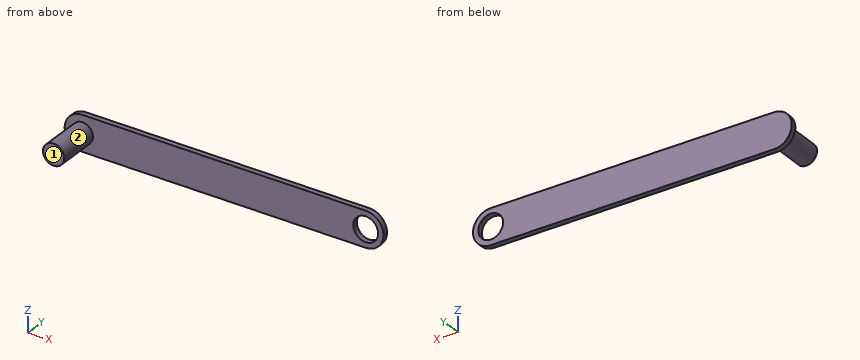
```python
from build123d import *

# Parameters (mm, degrees)
F0_R     = 3.5
F1_DEPTH = 1.5
F2_R     = 3
F3_DEPTH = 12


with BuildPart() as f1:
    # F0 (on Front) → F1 (new body)
    with BuildSketch(Plane.XZ):
        with BuildLine():
            Line((80, 5), (0, 5))
            ThreePointArc((0, 5), (-5, 0), (0, -5))
            Line((0, -5), (80, -5))
            ThreePointArc((80, -5), (85, 0), (80, 5))
        make_face()
        with Locations((80, 0)):
            Circle(F0_R, mode=Mode.SUBTRACT)
    extrude(amount=F1_DEPTH)

    # F2 (on face) → F3 (join)
    with BuildSketch(Plane.XZ.offset(1.5)):
        Circle(F2_R)
    extrude(amount=F3_DEPTH)


solid = f1.part
```
Source: CAD feature listing. Evaluate the final solid. Frame: model axes, mm. Face numbers are marked on the shaded views. Give positions to 0.01 mm unless a question says otherwise; leave off trailing zeros. Order: outer loops, then holes, each group sorted by start corner. A loop starts at its lowest first (then second) coordinate and runs counter-clockwise, first axis right, second up. Notation, with made-up numbers: (23.5, 77.5) -> (68.5, 77.5) arc R24 ccw to (68.5, 91.5) -> close; hole circle Ø8 at (-3.5, -39.75). An arc over 180 degrees is marked (long way). Use a Markdown table: item, result.
Q1. Section A-A (z = 0). Return the cut outline in (x, y), and give its area (4 significant figures).
A:
| item | result |
|---|---|
| outline | (-5, -1.5) -> (-3, -1.5) -> (-3, -13.5) -> (3, -13.5) -> (3, -1.5) -> (76.5, -1.5) -> (76.5, 0) -> (-5, 0) -> close; (83.5, -1.5) -> (85, -1.5) -> (85, 0) -> (83.5, 0) -> close |
| area | 196.5 mm^2 |
Q2. Section B-B (x = 2). Return the cut outline in (y, z).
A:
| item | result |
|---|---|
| outline | (-13.5, -2.24) -> (-1.5, -2.24) -> (-1.5, -5) -> (0, -5) -> (0, 5) -> (-1.5, 5) -> (-1.5, 2.24) -> (-13.5, 2.24) -> close |
Q3. Material intervals for line 1 (Z direction, x = 80, y = -0.8); line 2 (Y direction, x = 10, z = -2); line 3 (X direction, y = -1, z = -3.75), sorted ascending. Write a range as [from, to].
A:
| item | result |
|---|---|
| line 1 | [-5, -3.5], [3.5, 5] |
| line 2 | [-1.5, 0] |
| line 3 | [-3.31, 83.31] |
Q4. Pull-direction query (Z, two-part tool) for the marked faces 1 and 2; classes: +Z half, -Z half, draft (parallel to the pull), parting line (faces both ways), or undercut.
A:
| item | result |
|---|---|
| face 1 | draft |
| face 2 | parting line |
Q5. First-contact query: P1, Ø6, axis at x = 42.5, z = 4, coming from the -Y side; P2, Ø1, axis at x = 73.5, y = -2.5, coming from the +Z side. Flat tips, straight axial feed; report the tip coordinate or a pass-through.
A:
| item | result |
|---|---|
| P1 | y = -1.5 |
| P2 | through |
Q6. Section D-D (x = 43). Return the cut outline in (y, z), and give its area (3 significant figures).
A:
| item | result |
|---|---|
| outline | (-1.5, -5) -> (0, -5) -> (0, 5) -> (-1.5, 5) -> close |
| area | 15.0 mm^2 |
Q7. Section C-C (y = -3.5). Return the cut outline in (x, z), and give its area (3 significant figures).
A:
| item | result |
|---|---|
| outline | circle Ø6 at (0, 0) |
| area | 28.3 mm^2 |
